Geometry: see drawing. Coordinates: mm, zero at the bounding-box minimum. A direction names the side the tool comes from. Round coordinates to 2 decimals unless told otherwise and drop trailing zeros. Write each loop counter-clockwise with the first axis right and the second up, starting at its lowest first coordinate (ties: lowest second). Pieces come first, ordered by that corner, then holes. Notation, with made-up numbers: M 65,-2.5 L 84,-2.5 A21 cw 84,4.5 Z; hole C 9,-29.5 d9. An arc over 180 degrees is marked long. Write each question's results on one line, items separated by ' | '. Start each with the question number.
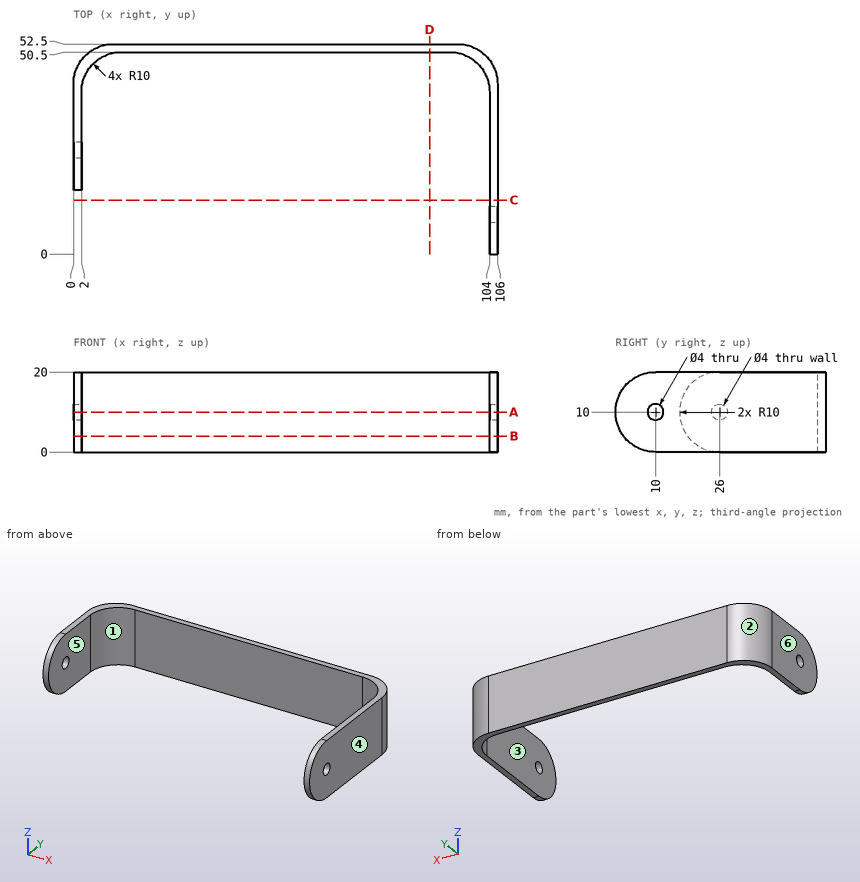
1. Cut plane D-D on x = 89. Output: boundary loops of the cut face in (y, z).
2. Cut plane A-A on z = 10. Output: boundary loops of the cut face in (x, y).
3. Access query for the marked faces 1 and 2. Directions: +Z, -Z, +X, -X, +Y, -Y. A direction counts if a zero-diameter tool reaches every point of the face in a straight line with its end or side. Return the directions, or none.
4. Cut plane B-B on z = 4. Output: boundary loops of the cut face in (x, y).
5. Draft query along X for the marked faces 3, 4, 5 and 6. Return one class per face: +X half, -X half, draft (parallel to the pull), parting line (faces both ways), or undercut.
6. Line query: L1, parallel to X at y = 34.5, z = 14; L2, parallel to X at y = 5.5, z = 18.75; L3, parallel to X at y = 46.5, z = 12.5. Output: solid intervals per line, ascending. Write a range as from..to.
7. Contact query for a flat-ended pin moving along its axis: P1, Ø10, axis at x = 50, z = 10, coming from the -Y side. Output: stop coordinate, or through.
8. Cut plane C-C on y = 13.5. Output: boundary loops of the cut face in (x, z).
Answers follow:
1) outline: M 50.5,0 L 52.5,0 L 52.5,20 L 50.5,20 Z
2) outline: M 0,16 L 2,16 L 2,24 L 0,24 Z; M 0,28 L 2,28 L 2,40.5 A10 cw 12,50.5 L 94,50.5 A10 cw 104,40.5 L 104,12 L 106,12 L 106,42.5 A10 ccw 96,52.5 L 10,52.5 A10 ccw 0,42.5 Z; M 104,0 L 106,0 L 106,8 L 104,8 Z
3) face 1: +Z, -Z, -Y | face 2: +Z, -Z, -X, +Y
4) outline: M 0,18 L 2,18 L 2,40.5 A10 cw 12,50.5 L 94,50.5 A10 cw 104,40.5 L 104,2 L 106,2 L 106,42.5 A10 ccw 96,52.5 L 10,52.5 A10 ccw 0,42.5 Z
5) face 3: undercut | face 4: +X half | face 5: undercut | face 6: -X half
6) L1: x = 0..2, 104..106 | L2: x = 104..106 | L3: x = 0.83..4, 102..105.17
7) P1: stops at y = 50.5
8) outline: M 104,0 L 106,0 L 106,20 L 104,20 Z
